Could you check a few things on this model? Use its own coordinates, in mm. Face numbers are marked on the shaded views. A direction names the side the tool comes from. Give positions to 0.01 mm unless a question says otherwise; leave off trailing zeros. Write each loop counter-clockwise with the first axis right and the second up, starting at its lowest first coordinate (ties: lowest second). Pieces come first, ordered by that corner, then holes. Notation, with made-up numbers: (-22.5, 5.25) - (4.5, 5.25) arc R34 ccw to (4.5, 44.25) - close; hole circle Ø9 at (-1, 64.25). An arc over 180 degrees is marked (long way). Answer in a Markdown table with one row per item.
Autodesk Inventor part; units mm, degrees
ref_plane "Work Plane1" through (-8.1491, -81.1802, -17.0906) normal (0, -1, 0) x (0.7071068, 0, 0.7071068)
ref_plane "YZ Plane" through (0, 0, 0) normal (1, 0, 0) x (0, 1, 0)
ref_plane "XZ Plane" through (0, 0, 0) normal (0, 1, 0) x (-1, 0, 0)
sketch "Sketch1" plane through (0, 0, 0) normal (0, 0, 1) x (1, 0, 0)
  line L0 (8.404, 3) -> (8.404, -46.6888)
  line L1 (6.389, 0.2) -> (6.389, -55.1706)
  line L2 (7.404, -64.4706) -> (6.389, -64.4706)
  line L3 (6.389, -64.4706) -> (6.389, -78.3802)
  line L4 (-3.1786, -78.3802) -> (6.389, -78.3802)
  line L5 (-3.1786, -78.3802) -> (-3.1786, -81.1802)
  line L6 (8.404, -81.1802) -> (-3.1786, -81.1802)
  line L7 (8.404, -65.4706) -> (8.404, -81.1802)
  line L8 (8.604, -55.6706) -> (6.189, -55.6706)
  line L9 (6.189, -55.6706) -> (6.189, 0)
  line L10 (6.189, 0) -> (-3.3786, 0)
  line L11 (-3.3786, 0) -> (-3.3786, 3.2)
  line L12 (-3.3786, 3.2) -> (8.604, 3.2)
  line L13 (8.604, 3.2) -> (8.604, -55.6706)
  line L14 (8.604, -81.3802) -> (-3.3786, -81.3802)
  line L15 (-3.3786, -81.3802) -> (-3.3786, -78.1802)
  line L16 (-3.3786, -78.1802) -> (6.189, -78.1802)
  line L17 (6.189, -78.1802) -> (6.189, -64.2706)
  line L18 (6.189, -64.2706) -> (8.604, -64.2706)
  line L19 (8.604, -64.2706) -> (8.604, -81.3802)
  line L20 (13.604, -60.6706) -> (1.189, -60.6706)
  line L21 (1.189, -60.6706) -> (1.189, -5)
  line L22 (1.189, -5) -> (-8.3786, -5)
  line L23 (-8.3786, -5) -> (-8.3786, 8.2)
  line L24 (-8.3786, 8.2) -> (13.604, 8.2)
  line L25 (13.604, 8.2) -> (13.604, -60.6706)
  circle A0 centre (13.604, -26.2353) radius 5
  line L26 (18.604, -65.6706) -> (-3.811, -65.6706)
  line L27 (-3.811, -65.6706) -> (-3.811, -10)
  line L28 (-3.811, -10) -> (-13.3786, -10)
  line L29 (-13.3786, -10) -> (-13.3786, 13.2)
  line L30 (-13.3786, 13.2) -> (18.604, 13.2)
  line L31 (18.604, 13.2) -> (18.604, -65.6706)
  circle A1 centre (13.604, -26.2353) radius 1.6
  circle A2 centre (13.604, -26.2353) radius 30.3549
  circle A3 centre (13.604, -26.2353) radius 38.3626
  line L32 (8.604, -55.6706) -> (8.604, -56.1756)
  line L33 (6.189, -64.2706) -> (6.189, -63.8744)
  line L34 (6.189, -63.8744) -> (18.604, -63.8744)
  line L35 (6.189, -63.8744) -> (18.604, -63.8744) construction
  line L36 (8.604, -55.6706) -> (1.189, -55.6706)
  line L37 (1.189, -55.6706) -> (1.189, -63.8744)
  line L38 (1.189, -63.8744) -> (18.604, -63.8744)
  line L39 (1.189, -62.5334) -> (18.604, -62.5334)
  line L40 (1.189, -62.5334) -> (18.604, -62.5334) construction
  line L41 (6.389, -55.1706) -> (12.3969, -55.1706)
  line L42 (12.604, -54.9635) -> (12.3969, -55.1706)
  line L43 (12.604, -46.8959) -> (12.604, -54.9635)
  line L44 (12.3969, -46.6888) -> (12.604, -46.8959)
  line L45 (8.404, -46.6888) -> (12.3969, -46.6888)
  line L46 (-3.1786, 3) -> (8.404, 3)
  line L47 (-3.1786, 0.2) -> (-3.1786, 3)
  line L48 (-3.1786, 0.2) -> (6.389, 0.2)
  circle A4 centre (9.4965, -50.9297) radius 1.5
  line L49 (7.404, -64.4706) -> (8.404, -65.4706)
  point P0 (0, 0)
  point P1 (8.604, -26.2353)
  point P2 (18.604, -26.2353)
  dimension "d0" = 0.2
  dimension "d1" = 0.2
  dimension "d2" = 5
  dimension "d3" = 5
  dimension "d4" = 3.2
  dimension "d5" = 0
  dimension "d6" = 0
extrude "Extrusion1" add sketch "Sketch1" along normal blind 2.5 contours L45 L44 L43 L42 L41 L13 A4 | L13 A0 L25 A2 L32 L41 L42 L43 L44 L45 | A0 L25 A1 | A4 L13 | A0 L25 A1 | A0 L31 A2 L25 | A2 L31 L39 L37 L20 L25 | L25 L20 L21 L36 A2 | L8 L32 A2 picked at (9.3865, -50.8083) picked at (16.7555, -47.8971)
sketch "Sketch2" plane through (1.189, -62.5334, 0) normal (0, -1, 0) x (1, 0, 0)
  line L0 (-0.8528, -0.0858) -> (2.6827, 3.4497)
  line L1 (-0.7114, -0.2272) -> (2.8241, 3.3083)
  line L2 (0, 2.5) -> (17.415, 2.5)
  line L3 (0, 0) -> (0, 2.5)
  point P0 (-1.189, 0)
  point P1 (0, 0.4842)
  point P2 (2.0158, 2.5)
  dimension "d9" = 0.2
extrude "Extrusion2" cut sketch "Sketch2" against normal through all
sketch "Sketch4" plane through (1.189, -62.5334, 0) normal (0, -1, 0) x (1, 0, 0)
  line L0 (2.0158, 2.5) -> (17.415, 2.5)
  line L1 (0, 0) -> (17.415, 0)
  line L2 (17.415, 0) -> (17.415, 2.5)
  line L3 (7.415, 0) -> (7.415, 2.5)
  point P0 (-1.189, 0)
ref_plane "Work Plane1" through (-8.1491, -81.1802, -17.0906) normal (0, -1, 0) x (0.7071068, 0, 0.7071068)
extrude "Extrusion3" add sketch "Sketch4" along normal up to surface (18.6468 mm away)
sketch "Sketch5" plane through (0, 0, 2.5) normal (0, 0, 1) x (1, 0, 0)
  line L0 (8.604, -26.2353) -> (8.604, -55.6706)
  circle A0 centre (13.604, -26.2353) radius 1.6
  circle A1 centre (13.604, -26.2353) radius 29.857
  line L1 (8.604, -26.2353) -> (8.604, -55.6706)
  line L2 (8.604, -55.6706) -> (12.604, -55.6706)
  line L3 (8.604, -55.6706) -> (12.604, -55.6706) construction
  line L4 (12.604, -55.6706) -> (8.604, -55.6706)
  line L5 (8.604, -55.6706) -> (8.604, -51.6706)
  line L6 (8.604, -51.6706) -> (12.604, -51.6706)
  line L7 (12.604, -51.6706) -> (12.604, -55.6706)
  line L8 (12.604, -51.6706) -> (8.604, -51.6706)
  line L9 (8.604, -51.6706) -> (8.604, -47.6706)
  line L10 (8.604, -47.6706) -> (12.604, -47.6706)
  line L11 (12.604, -47.6706) -> (12.604, -51.6706)
  line L12 (12.604, -47.6706) -> (8.604, -47.6706)
  line L13 (8.604, -47.6706) -> (8.604, -46.6706)
  line L14 (8.604, -46.6706) -> (12.604, -46.6706)
  line L15 (12.604, -46.6706) -> (12.604, -47.6706)
  circle A2 centre (13.604, -26.2353) radius 20.4598
  circle A3 centre (13.604, -26.2353) radius 19.9598
  line L16 (12.604, -55.6706) -> (13.104, -55.6706)
  line L17 (13.104, -55.6706) -> (13.104, -46.1888)
  line L18 (13.104, -46.1888) -> (8.604, -46.1888)
  point P0 (0, 0)
  dimension "d22" = 0.5
  dimension "d14" = 4
  dimension "d15" = 0
  dimension "d16" = 4
  dimension "d17" = 4
  dimension "d18" = 4
  dimension "d19" = 4
  dimension "d20" = 4
  dimension "d21" = 1
  dimension "d23" = 0.5
  dimension "d24" = 90
  dimension "d25" = 90
extrude "Extrusion4" cut sketch "Sketch5" against normal blind 10 contours L18 A2 L14 L0 | L14 L15 L10 L0 | L18 L17 A2 | L10 L11 L6 L0 | A2 L17 L16 L7 L11 L15 | L6 L7 L2 L0
chamfer "Chamfer1" distance 0.5 angle 45 3 edges at (8.604, -46.1888, 1.25) (13.104, -46.1888, 1.25) (13.104, -55.6706, 1.25)
sketch "Sketch6" plane through (0, 0, 2.5) normal (0, 0, 1) x (1, 0, 0)
  line L0 (18.604, -26.2353) -> (18.604, -81.1802)
  line L1 (8.604, -62.5334) -> (8.604, -81.1802)
  line L2 (15.604, -26.2353) -> (15.604, -81.1802)
  line L3 (11.604, -62.5334) -> (11.604, -81.1802)
  line L4 (11.604, -62.5334) -> (15.604, -62.5334)
  line L5 (15.604, -62.5334) -> (15.604, -81.1802)
  line L6 (15.604, -81.1802) -> (11.604, -81.1802)
  line L7 (11.604, -81.1802) -> (11.604, -62.5334)
  point P0 (0, 0)
  dimension "d31" = 3
  dimension "d32" = 3
extrude "Extrusion5" add sketch "Sketch6" along normal blind 6
chamfer "Chamfer2" distance 2 angle 45 2 edges at (11.604, -71.8568, 2.5) (15.604, -71.8568, 2.5)
sketch "Sketch7" plane through (0, 0, 2.5) normal (0, 0, 1) x (1, 0, 0)
  line L0 (18.604, -26.2353) -> (18.604, -81.1802)
  line L1 (9.104, -46.1888) -> (12.604, -46.1888)
  line L2 (9.104, -44.1888) -> (12.604, -44.1888)
  line L3 (18.604, -44.1888) -> (15.604, -44.1888)
  line L4 (15.604, -44.1888) -> (15.604, -37.1888)
  line L5 (15.604, -37.1888) -> (18.604, -37.1888)
  line L6 (18.604, -37.1888) -> (18.604, -44.1888)
  point P0 (0, 0)
  dimension "d38" = 2
  dimension "d39" = 3
  dimension "d40" = 7
extrude "Extrusion6" cut sketch "Sketch7" against normal blind 6
sketch "Sketch9" plane through (1.189, -62.5334, 0) normal (0, -1, 0) x (1, 0, 0)
  line L0 (2.0158, 2.5) -> (7.415, 2.5)
  line L1 (2.0158, 2.5) -> (0, 0.4842)
  line L2 (7.415, 0) -> (7.415, 2.5)
  line L3 (7.415, 2.5) -> (7.415, 5.5)
  line L4 (7.415, 2.5) -> (10.415, 2.5) construction
  line L5 (0, 0.4842) -> (5.0158, 5.5)
  line L6 (17.415, 2.5) -> (17.415, 0)
  line L7 (5.0158, 5.5) -> (17.415, 5.5)
  line L8 (5.0158, 5.5) -> (17.415, 5.5) construction
  line L9 (17.415, 5.5) -> (17.415, 2.5)
  line L10 (17.415, 2.5) -> (7.415, 2.5)
  point P0 (-1.189, 0)
  dimension "d43" = 3
  dimension "d44" = 90
  dimension "d45" = 0
extrude "Extrusion7" add sketch "Sketch9" against normal blind 3
chamfer "Chamfer3" distance 2 angle 45 1 edges at (18.604, -59.5334, 4)
chamfer "Chamfer4" distance 3 angle 45 1 edges at (13.604, -62.5334, 5.5)
properties part number "LatchLock_3DPrint"
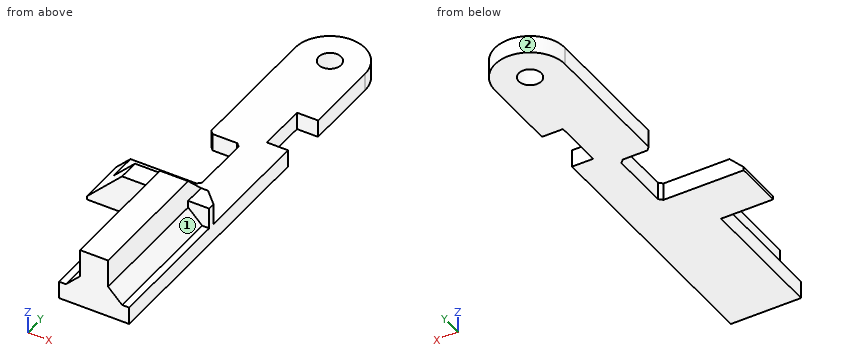
1) On a 3-axis mill with a long thin cutter (end or side, diameter ignored), from which of +Z, -Z, +X, -X, +Y, -Y can I reach the whole of each face in a straight line? I mean the marked faces 1 and 2. Say none if no direction works.
Check values:
| item | result |
|---|---|
| face 1 | +Z, +X, -Y |
| face 2 | +Z, -Z, +Y |
2) If I drill on line 1 (Y direction, x = 14.25, z = 4.75); line 2 (X direction, y = -70, z = 2); line 3 (Z direction, x = 14.5, y = -39), over which ranges is the centre line in solid material (lowest first)?
Check values:
| item | result |
|---|---|
| line 1 | y = -81.18 to -59.53 |
| line 2 | x = 8.6 to 18.6 |
| line 3 | z = 0 to 2.5 |
3) Will these pins go through, and if not, where does the flat tip stop? P1, Ø3, axis at x = 5, z = 3.5, coming from the -Y side; P2, Ø0.8, axis at y = -51, z = 0.5, coming from the -X side; P3, Ø5, axis at x = 12, z = 5.5, coming from the +Y side; P4, Ø3, axis at x = 13.6, y = -26.24, coming from the +Z side.
Check values:
| item | result |
|---|---|
| P1 | stops at y = -62.53 |
| P2 | stops at x = 13.1 |
| P3 | stops at y = -59.53 |
| P4 | passes through |
4) Imagine slicing it at B-B (x = 10.5). List the corners of the cut face in (y, z) for me, then the cut area to 3 significant figures.
Check values:
| item | result |
|---|---|
| outline | (-81.18, 0) - (-55.67, 0) - (-55.67, 2.5) - (-59.53, 2.5) - (-59.53, 5.5) - (-62.53, 5.5) - (-62.53, 3.4) - (-81.18, 3.4) - close; (-46.19, 0) - (-22.32, 0) - (-22.32, 2.5) - (-46.19, 2.5) - close |
| area | 149 mm2 |
5) Imagine slicing it at D-D (x = 4.5). List the corners of the cut face in (y, z) for me, then the cut area to 3 significant figures.
Check values:
| item | result |
|---|---|
| outline | (-62.53, 0) - (-55.67, 0) - (-55.67, 2.5) - (-59.53, 2.5) - (-59.53, 3.8) - (-62.53, 3.8) - close |
| area | 21.0 mm2 |
6) Imagine slicing it at A-A (y = -67.5). List the corners of the cut face in (x, z) for me, then the cut area to 3 significant figures.
Check values:
| item | result |
|---|---|
| outline | (8.6, 0) - (18.6, 0) - (18.6, 2.5) - (17.6, 2.5) - (15.6, 4.5) - (15.6, 8.5) - (11.6, 8.5) - (11.6, 4.5) - (9.6, 2.5) - (8.6, 2.5) - close |
| area | 53.0 mm2 |
7) Imagine slicing it at C-C (z = 1.25). List the corners of the cut face in (x, y) for me, then the cut area to 3 significant figures.
Check values:
| item | result |
|---|---|
| outline | (1.95, -62.53) - (8.6, -62.53) - (8.6, -81.18) - (18.6, -81.18) - (18.6, -44.19) - (15.6, -44.19) - (15.6, -37.19) - (18.6, -37.19) - (18.6, -26.24) arc R5 ccw to (8.6, -26.24) - (8.6, -45.69) - (9.1, -46.19) - (12.6, -46.19) - (13.1, -46.69) - (13.1, -55.17) - (12.6, -55.67) - (1.95, -55.67) - close; hole circle Ø3.2 at (13.6, -26.24) |
| area | 563 mm2 |
